```python
from build123d import *

# Parameters (mm, degrees)
PAD_DEPTH            = 10
POCKET_DEPTH         = 0.001
POCKET_DEPTH_BACK    = 10.001
POCKET001_DEPTH      = 0.001
POCKET001_DEPTH_BACK = 10.001
POCKET002_DEPTH      = 0.001
POCKET002_DEPTH_BACK = 10.001
POCKET003_DEPTH      = 0.001
POCKET003_DEPTH_BACK = 10.001
POCKET004_DEPTH      = 0.001
POCKET004_DEPTH_BACK = 10.001
POCKET005_DEPTH      = 0.001
POCKET005_DEPTH_BACK = 10.001
POCKET006_DEPTH      = 0.001
POCKET006_DEPTH_BACK = 10.001
POCKET007_DEPTH      = 0.001
POCKET007_DEPTH_BACK = 10.001


with BuildPart() as part:
    # Sketch → Pad (new body)
    with BuildSketch(Plane.XY):
        Polygon((-24.869964, 16.395561), (-11.340966, 16.395561), (-11.340966, 23.768572), (8.37961, 23.768572), (8.37961, 16.040237), (21.881983, 16.040237), (21.881983, -23.94381), (6.594811, -23.94381), (6.594811, -20.773636), (-9.572513, -20.773636), (-9.572513, -24.250378), (-24.869964, -24.250378), align=None)
    extrude(amount=PAD_DEPTH)

    # Sketch001 → Pocket (cut, two sides)
    with BuildSketch(Plane.XY) as pocket_sk:
        Polygon((7.042854, 14.493185), (7.042854, -0.376181), (7.60472, -0.376181), (7.60472, -0.938048), (10.529679, -0.938048), (10.529679, -0.392844), (20.320467, -0.392844), (20.320467, 4.433404), (20.320467, 12.107393), (20.320467, 14.493185), (11.347224, 14.493185), (7.737097, 14.493185), align=None)
    extrude(amount=-POCKET_DEPTH, mode=Mode.SUBTRACT)
    extrude(pocket_sk.sketch, amount=POCKET_DEPTH_BACK, mode=Mode.SUBTRACT)

    # Sketch002 → Pocket001 (cut, two sides)
    with BuildSketch(Plane.XY) as pocket001_sk:
        Polygon((6.562266, -8.697514), (6.562266, 17.730482), (6.562266, 20.972402), (6.562266, 22.205465), (4.247283, 22.205465), (4.247283, 23.77135), (-7.208705, 23.77135), (-7.208705, 22.236126), (-9.579967, 22.236126), (-9.579967, 20.501596), (-9.579967, 17.725863), (-9.579967, -8.859713), (-5.78053, -8.859713), (-5.78053, -9.246999), (-1.996924, -9.246999), (-1.996924, -8.697514), align=None)
    extrude(amount=-POCKET001_DEPTH, mode=Mode.SUBTRACT)
    extrude(pocket001_sk.sketch, amount=POCKET001_DEPTH_BACK, mode=Mode.SUBTRACT)

    # Sketch003 → Pocket002 (cut, two sides)
    with BuildSketch(Plane.XY) as pocket002_sk:
        Polygon((-9.555696, 14.58253), (-11.251103, 14.58253), (-14.140704, 14.58253), (-23.244276, 14.58253), (-23.244276, 10.916287), (-23.244276, 3.175509), (-23.244276, -3.024841), (-14.543381, -3.024841), (-14.543381, -0.542157), (-13.913779, -0.542157), (-13.913779, -3.319152), (-9.555696, -3.319152), align=None)
    extrude(amount=-POCKET002_DEPTH, mode=Mode.SUBTRACT)
    extrude(pocket002_sk.sketch, amount=POCKET002_DEPTH_BACK, mode=Mode.SUBTRACT)

    # Sketch004 → Pocket003 (cut, two sides)
    with BuildSketch(Plane.XY) as pocket003_sk:
        Polygon((-23.265747, -7.57667), (-23.265747, -22.274162), (-20.999838, -22.274162), (-13.232408, -22.274162), (-11.332763, -22.274162), (-11.332763, -18.95647), (-9.916094, -18.95647), (-9.916094, -7.509449), (-10.598124, -7.509449), (-10.598124, -6.945273), (-9.384972, -6.945273), (-9.384972, -0.656561), (-13.872682, -0.656561), (-13.872682, -3.571327), (-23.414576, -3.571327), (-23.414576, -7.059722), (-14.509603, -7.059722), (-14.509603, -6.304652), (-13.875799, -6.304652), (-13.875799, -7.078746), (-13.37953, -7.078746), (-13.37953, -7.57667), align=None)
    extrude(amount=-POCKET003_DEPTH, mode=Mode.SUBTRACT)
    extrude(pocket003_sk.sketch, amount=POCKET003_DEPTH_BACK, mode=Mode.SUBTRACT)

    # Sketch005 → Pocket004 (cut, two sides)
    with BuildSketch(Plane.XY) as pocket004_sk:
        Polygon((-9.459572, -9.286458), (-9.459572, -18.99835), (-6.993228, -18.99835), (-2.81149, -18.99835), (-1.42501, -18.99835), (-1.42501, -9.292158), (-1.95218, -9.292158), (-1.95218, -8.499968), (-5.901244, -8.499968), (-5.901244, -9.286458), align=None)
    extrude(amount=-POCKET004_DEPTH, mode=Mode.SUBTRACT)
    extrude(pocket004_sk.sketch, amount=POCKET004_DEPTH_BACK, mode=Mode.SUBTRACT)

    # Sketch006 → Pocket005 (cut, two sides)
    with BuildSketch(Plane.XY) as pocket005_sk:
        Polygon((-1.187414, -9.325391), (-1.187414, -19.042973), (3.81931, -19.042973), (6.650182, -19.042973), (6.650182, -9.325391), align=None)
    extrude(amount=-POCKET005_DEPTH, mode=Mode.SUBTRACT)
    extrude(pocket005_sk.sketch, amount=POCKET005_DEPTH_BACK, mode=Mode.SUBTRACT)

    # Sketch007 → Pocket006 (cut, two sides)
    with BuildSketch(Plane.XY) as pocket006_sk:
        Polygon((6.904032, -6.522334), (6.904032, -7.023237), (7.502099, -7.023237), (7.502099, -7.587341), (6.984618, -7.587341), (6.984618, -19.001835), (8.102534, -19.001835), (8.102534, -22.300638), (10.341199, -22.300638), (18.38561, -22.300638), (20.463644, -22.300638), (20.463644, -8.397645), (10.979427, -8.397645), (10.979427, -7.547909), (10.426148, -7.547909), (10.426148, -7.063529), (10.909175, -7.063529), (10.909175, -6.522334), align=None)
    extrude(amount=-POCKET006_DEPTH, mode=Mode.SUBTRACT)
    extrude(pocket006_sk.sketch, amount=POCKET006_DEPTH_BACK, mode=Mode.SUBTRACT)

    # Sketch008 → Pocket007 (cut, two sides)
    with BuildSketch(Plane.XY) as pocket007_sk:
        Polygon((11.501872, -3.733678), (11.501872, -7.893655), (20.367885, -7.893655), (20.367885, -5.953888), (20.367885, -2.59785), (20.367885, -0.882918), (11.555678, -0.882918), (11.555678, -1.383317), (10.838286, -1.383317), (10.838286, -0.96668), (6.526137, -0.96668), (6.526137, -6.505466), (10.874155, -6.505466), (10.874155, -3.715743), align=None)
    extrude(amount=-POCKET007_DEPTH, mode=Mode.SUBTRACT)
    extrude(pocket007_sk.sketch, amount=POCKET007_DEPTH_BACK, mode=Mode.SUBTRACT)


solid = part.part
```
Check sheet for the modelled part. Datum: model origin and axes. Units: mm. A direction names the side the tool comes from. Coordinates: 2 decimals unless noted, no trailing zeros. Order: outer loops, then holes, each group sorted by start corner. A loop starts at its lowest first (then second) coordinate and runs counter-clockwise, first axis right, second up. Notation, with made-up numbers: (28.25, 48.5) -> (64.25, 48.5) arc R20 cw to (64.25, 84.5) -> close; hole circle Ø11 at (-23, 55.25). An arc over 180 degrees is marked (long way). Write each question's results on one line, items separated by ' | '. Start each with the question number.
1) Material ranges on line 1 along Y through (x, z) = (-20, 6.5); line 2 along X through (y, z) = (8.5, 4); line 3 along X through (y, z) = (-14, 6.25), recorded low to high.
2) Section check A-A (x = -16). Enter the section's corners in (y, z), and give its area (3 significant figures).
3) Draft check along Y on faces 1 (the face through (15, 16.04, 5)), 2 (the face through (10.874, -5, 5)), 3 (the face through (6.595, -22, 5)). Enter one of: pulls with the +Y half, pulls with the -Y half, needs draft (parallel to the pull), parting line crosses it, or undercut.
4) Section check D-D (x = 19). Enter the section's corners in (y, z), and give its area (3 significant figures).
5) Section check B-B (y = 19). Enter the section's corners in (x, z), and give its area (3 significant figures).
6) Set-up check for faces 4 (the face through (11.502, -6, 5)), 5 (the face through (-24.87, -4, 5)): record each of +Z, -Z, +X, -X, +Y, -Y from which the full face is reachable in a straight line by a thin tool's end or side.
7) Section check C-C (y = 13). Enter the section's corners in (x, z).
Checked values:
1) line 1: -24.25 to -22.27, -7.58 to -7.06, -3.57 to -3.02, 14.58 to 16.4 | line 2: -24.87 to -23.24, 6.56 to 7.04, 20.32 to 21.88 | line 3: -24.87 to -23.27, -9.92 to -9.46, -1.43 to -1.19, 6.65 to 6.98, 20.46 to 21.88
2) outline: (-24.25, 0) -> (-22.27, 0) -> (-22.27, 10) -> (-24.25, 10) -> close; (-7.58, 0) -> (-7.06, 0) -> (-7.06, 10) -> (-7.58, 10) -> close; (-3.57, 0) -> (-3.02, 0) -> (-3.02, 10) -> (-3.57, 10) -> close; (14.58, 0) -> (16.4, 0) -> (16.4, 10) -> (14.58, 10) -> close | area: 48.5 mm²
3) face 1: pulls with the +Y half | face 2: undercut | face 3: needs draft
4) outline: (-23.94, 0) -> (-22.3, 0) -> (-22.3, 10) -> (-23.94, 10) -> close; (-8.4, 0) -> (-7.89, 0) -> (-7.89, 10) -> (-8.4, 10) -> close; (-0.88, 0) -> (-0.39, 0) -> (-0.39, 10) -> (-0.88, 10) -> close; (14.49, 0) -> (16.04, 0) -> (16.04, 10) -> (14.49, 10) -> close | area: 41.8 mm²
5) outline: (-11.34, 0) -> (-9.58, 0) -> (-9.58, 10) -> (-11.34, 10) -> close; (6.56, 0) -> (8.38, 0) -> (8.38, 10) -> (6.56, 10) -> close | area: 35.8 mm²
6) face 4: +Z, -Z | face 5: +Z, -Z, -X, +Y, -Y
7) outline: (-24.87, 0) -> (-23.24, 0) -> (-23.24, 10) -> (-24.87, 10) -> close; (6.56, 0) -> (7.04, 0) -> (7.04, 10) -> (6.56, 10) -> close; (20.32, 0) -> (21.88, 0) -> (21.88, 10) -> (20.32, 10) -> close
